Work out the finished part from the listing and answer in its coordinate system (mm). A direction names the side the tool comes from. Round coordinates to 2 decimals unless told otherwise and drop trailing zeros. Write each loop counter-clockwise with the first axis right and the second up, starting at its lowest first coordinate (ties: lowest second). Pieces come first, ordered by that corner, then holes. Notation, with made-up numbers: M -34.75,30 L -14.75,30 A12 cw -14.75,37 Z; hole C -39.75,-20 d6. An arc over 180 degrees is marked long. Answer in a Markdown table with one row per item.
```python
from build123d import *

# Parameters (mm, degrees)
POCKET_DEPTH         = 24.001
POCKET_DEPTH_BACK    = 0.001
SKETCH004_W          = 40
SKETCH004_H          = 12
POCKET001_DEPTH      = 50.001
POCKET001_DEPTH_BACK = 0.001


with BuildPart() as part:
    # AdditivePipe: sweep along a path in Sketch
    with BuildLine(Plane.YZ) as additivepipe_path:
        Line((0, 0), (20, 0))
        Line((20, 0), (50, -12))
    # Sketch001 → AdditivePipe (sweep)
    with BuildSketch(Plane.XZ):
        Polygon((-20, 6), (-20, -6), (20, -6), (20, 6), (16, 6), (16, 3), (9, 3), (-9, 3), (-16, 3), (-16, 6), align=None)
    sweep(path=additivepipe_path.line)

    # Sketch003 → Pocket (cut, two sides)
    with BuildSketch(Plane(origin=(0, 0, 6), x_dir=(-1, 0, 0), z_dir=(0, 0, 1))) as pocket_sk:
        with BuildLine():
            Line((-4.5, 0), (4.5, 0))
            Line((4.5, 0), (4.5, -7))
            ThreePointArc((-4.5, -7), (0, -19.361903), (4.5, -7))
            Line((-4.5, 0), (-4.5, -7))
        make_face()
    extrude(amount=-POCKET_DEPTH, mode=Mode.SUBTRACT)
    extrude(pocket_sk.sketch, amount=POCKET_DEPTH_BACK, mode=Mode.SUBTRACT)

    # Sketch004 → Pocket001 (cut, two sides)
    with BuildSketch(Plane.XZ) as pocket001_sk:
        with Locations((0, -12)):
            Rectangle(SKETCH004_W, SKETCH004_H)
    extrude(amount=-POCKET001_DEPTH, mode=Mode.SUBTRACT)
    extrude(pocket001_sk.sketch, amount=POCKET001_DEPTH_BACK, mode=Mode.SUBTRACT)


solid = part.part
```
1. A tool of negligible diameter and unlimited length cuts with its end or side. For faces 1 (the flat face through (-4.5, 3, -1)), 2 (the cylindrical face through (0.239, 19.358, -1.437)), 3 (the flat face through (0.224, 31.407, -1.563)), from which of +Z, -Z, +X, -X, +Y, -Y can it reach the whole face along a straight path? Write none if from no direction.
Calculated:
| item | result |
|---|---|
| face 1 | +Z, -Z, -Y |
| face 2 | +Z, -Z |
| face 3 | +Z, +Y |
2. The part is cut by section D-D (x = 0). Determine the outline of the cut face in (y, z), plus the area to 3 significant figures.
Calculated:
| item | result |
|---|---|
| outline | M 19.36,-6 L 42.5,-6 L 20,3 L 19.36,3 Z |
| area | 107 mm² |
3. Consider line 1 along X through (y, z) = (9, 3.75); line 2 along Z through (x, y) = (-5.5, 4.5); line 3 along X through (y, z) = (15.5, 0.25). Determine where each line is inside the solid, lowest interval first. Write a range as from..to.
Calculated:
| item | result |
|---|---|
| line 1 | x = -20..-16, 16..20 |
| line 2 | z = -6..3 |
| line 3 | x = -20..-6.26, 6.26..20 |
4. The part is cut by section A-A (y = 46.5). Determine the outline of the cut face in (x, z), plus the area to 3 significant figures.
Calculated:
| item | result |
|---|---|
| outline | M -20,-6 L -16,-6 L -16,-4.6 L -20,-4.6 Z; M 16,-6 L 20,-6 L 20,-4.6 L 16,-4.6 Z |
| area | 11.2 mm² |
5. The part is cut by section B-B (z = -3). Determine the outline of the cut face in (x, y), plus the area to 3 significant figures.
Calculated:
| item | result |
|---|---|
| outline | M -20,0 L -4.5,0 L -4.5,7 A7 cw long 4.5,7 L 4.5,0 L 20,0 L 20,42.5 L 16,42.5 L 16,35 L -16,35 L -16,42.5 L -20,42.5 Z |
| area | 1,250 mm² |
6. Determine the mould class of faces 4 (the flat face through (-18, 10, 6)), 5 (the flat face through (-20, 20, -1)), 6 (the flat face through (7, 10, 3)) for opening direction X: released by +X, released by -X, zero draft, split by the parting line, or undercut.
Calculated:
| item | result |
|---|---|
| face 4 | zero draft |
| face 5 | released by -X |
| face 6 | undercut |
7. Given pin 1 (2 mm diameter, centred on x = -2.5, z = 1, fed in from +Y); pin 2 (5 mm diameter, centred on x = 0, z = -3, fed in from -Y); pin 3 (6 mm diameter, centred on x = 14.5, y = 33.5, fed in from +Z), each flat-ended and moving along its own axis, determine where each tip first touches the part or whether it passes through.
Calculated:
| item | result |
|---|---|
| pin 1 | stops at y = 27.5 |
| pin 2 | stops at y = 18.9 |
| pin 3 | stops at z = 1.64 |
8. The part is cut by section C-C (y = 37). Determine the outline of the cut face in (x, z), plus the area to 3 significant figures.
Calculated:
| item | result |
|---|---|
| outline | M -20,-6 L 20,-6 L 20,-0.8 L 16,-0.8 L 16,-3.8 L -16,-3.8 L -16,-0.8 L -20,-0.8 Z |
| area | 112 mm² |
